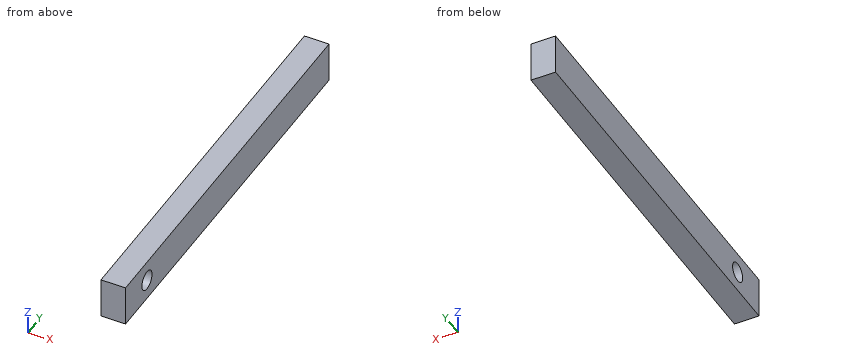
Autodesk Inventor part; units mm, degrees
ref_plane "YZ Plane" through (0, 0, 0) normal (1, 0, 0) x (0, 1, 0)
ref_plane "XZ Plane" through (0, 0, 0) normal (0, 1, 0) x (-1, 0, 0)
ref_plane "XY Plane" through (0, 0, 0) normal (0, 0, 1) x (1, 0, 0)
sketch "Sketch1" plane through (0, 0, 0) normal (0, 1, 0) x (-1, 0, 0)
  line L0 (-3, -5) -> (3, -5)
  line L1 (3, -5) -> (3, 5)
  line L2 (3, 5) -> (-3, 5)
  line L3 (-3, 5) -> (-3, -5)
  line L4 (-3, -5) -> (3, 5) construction
  line L5 (3, -5) -> (-3, 5) construction
  point P0 (0, 0)
  dimension "d0" = 6
  dimension "d1" = 10
extrude "Extrusion1" add sketch "Sketch1" along normal blind 95
sketch "Sketch2" plane through (-3, 0, -5) normal (-1, 0, 0) x (0, 0, 1)
  line L0 (0, 0) -> (10, 0)
  line L1 (0, 0) -> (0, 95)
  circle A0 centre (5, 10) radius 2.35
  line L2 (5, 0) -> (5, 20) construction
  dimension "d4" = 4.7
  dimension "d5" = 10
extrude "Extrusion2" cut sketch "Sketch2" against normal up to next
properties part number "WoodArm" material "Wood (Cherry)"
Work out the finished part from the listing and answer in its coordinate system (mm). Coordinates: 2 decimals unless noted, no trailing zeros. Write each loop counter-clockwise with the first axis right and the second up, starting at its lowest first coordinate (ties: lowest second). Pieces come first, ordered by that corner, then holes. Notation, with made-up numbers: M 12.25,20.25 L 53.25,20.25 A35 ccw 53.25,58.25 Z; hole C -2,16.5 d2. An arc over 180 degrees is marked long. Use one line per item in the form item = value. Start each with the question number.
1. This flat-tipped pin is pushed along its axis until it touches: P1, Ø3, axis at y = 10, z = 0, coming from the -X side. Where does it stop, or does it pass through?
2. The part is cut by section B-B (y = 10). Give the vertices of the cut face in (x, z), plus the area to 3 significant figures.
3. The part is cut by section C-C (x = 2.1). Give the vertices of the cut face in (y, z).
4. The part is cut by section A-A (z = 0). Give the vertices of the cut face in (x, y).
5. Straight lines are drawn through the part: probe 1 along Y at (x, z) = (1.7, 0); probe 2 along Y at (x, z) = (1, 2); probe 3 along Z at (x, y) = (2.5, 9). For each, find the intervals that lie inside material, in ascending order. Write a range as from..to.
Evaluation:
q1.P1 = through
q2.outline = M -3,-5 L 3,-5 L 3,-2.35 L -3,-2.35 Z; M -3,2.35 L 3,2.35 L 3,5 L -3,5 Z
q2.area = 31.8 mm^2
q3.outline = M 0,-5 L 95,-5 L 95,5 L 0,5 Z; hole C 10,0 d4.7
q4.outline = M -3,0 L 3,0 L 3,7.65 L -3,7.65 Z; M -3,12.35 L 3,12.35 L 3,95 L -3,95 Z
q5.probe_1 = 0..7.65, 12.35..95
q5.probe_2 = 0..8.77, 11.23..95
q5.probe_3 = -5..-2.13, 2.13..5
